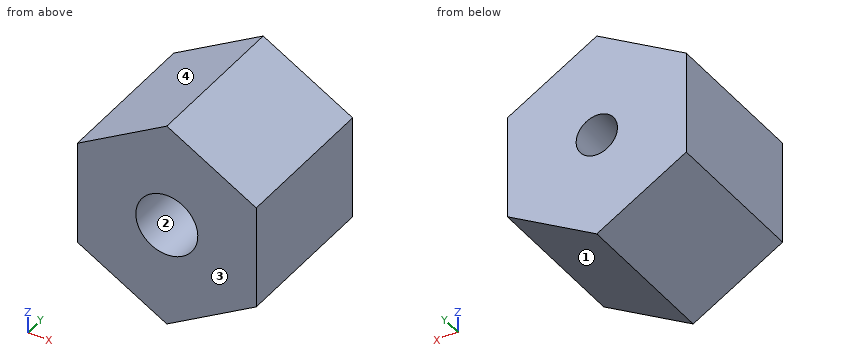
```python
from build123d import *

# Parameters (mm, degrees)
SKETCH2_R           = 2
BOSS_EXTRUDE1_DEPTH = 15
SKETCH2_4_R         = 3
CUT_EXTRUDE1_DEPTH  = 9


with BuildPart() as part:
    # Sketch2 → Boss-Extrude1 (new body)
    with BuildSketch(Plane(origin=(0, 0, 0), x_dir=(1, 0, 0), z_dir=(0, 1, 0))):
        Polygon((0, 10), (-8.660254038, 5), (-8.660254038, -5), (0, -10), (8.660254038, -5), (8.660254038, 5), align=None)
        with Locations(Location((0, 0, 0), (0, 0, 270))):
            Circle(SKETCH2_R, mode=Mode.SUBTRACT)
    extrude(amount=BOSS_EXTRUDE1_DEPTH)

    # Sketch2_4 → Cut-Extrude1 (cut)
    with BuildSketch(Plane(origin=(0, 0, 0), x_dir=(1, 0, 0), z_dir=(0, 1, 0))):
        with Locations(Location((0, 0, 0), (0, 0, 270))):
            Circle(SKETCH2_4_R)
    extrude(amount=CUT_EXTRUDE1_DEPTH, mode=Mode.SUBTRACT)


solid = part.part
```
Build history of the part. All positions in model axes, mm. Face numbers are marked on the shaded views. Coordinates: 2 decimals unless noted, no trailing zeros. Write each loop counter-clockwise with the first axis right and the second up, starting at its lowest first coordinate (ties: lowest second). Pieces come first, ordered by that corner, then holes.
1. Drop flat-ended pins along their axis: pin 1 (1.5 mm diameter, centred on x = -6.5, y = 6.5, fed in from -Z); pin 2 (3 mm diameter, centred on x = -3, y = 13, fed in from -Z); pin 3 (4 mm diameter, centred on x = -1, y = 7, fed in from +Z). Give the stop position or say it passes through.
Answer block:
pin 1: stops at z = -6.68
pin 2: stops at z = -9.13
pin 3: stops at z = 10
2. Drill centre lines: probe 1 along X at (y, z) = (10.9, 0); probe 2 along X at (y, z) = (2, 0); probe 3 along Z at (x, y) = (1.5, 11). Where is each one in solid material? Low to high.
Answer block:
probe 1: x = -8.66 to -2, 2 to 8.66
probe 2: x = -8.66 to -3, 3 to 8.66
probe 3: z = -9.13 to -1.32, 1.32 to 9.13
3. Pull direction X, two halves, no side cores. Call the marked faces 1, 2, 3 and 4: released by +X, released by -X, zero draft, split by the parting line, or undercut.
Answer block:
face 1: released by +X
face 2: undercut
face 3: zero draft
face 4: released by -X
4. Band-saw the part on D-D, the plane y = 7. Give the cut face in (x, z).
Answer block:
outline: (-8.66, -5) - (0, -10) - (8.66, -5) - (8.66, 5) - (0, 10) - (-8.66, 5) - close; hole circle Ø6 at (0, 0)
5. Band-saw the part on B-B, the plane z = 0. Give the cut face in (x, y).
Answer block:
outline: (-8.66, 0) - (-3, 0) - (-3, 9) - (-2, 9) - (-2, 15) - (-8.66, 15) - close; (2, 9) - (3, 9) - (3, 0) - (8.66, 0) - (8.66, 15) - (2, 15) - close
6. Band-saw the part on C-C, the plane x = -1.25. Give the cut face in (y, z), and give its area (3 significant figures).
Answer block:
outline: (0, -9.28) - (15, -9.28) - (15, -1.56) - (9, -1.56) - (9, -2.73) - (0, -2.73) - close; (0, 2.73) - (9, 2.73) - (9, 1.56) - (15, 1.56) - (15, 9.28) - (0, 9.28) - close
area: 211 mm2
7. Band-saw the part on A-A, the plane y = 11. Give the cut face in (x, z).
Answer block:
outline: (-8.66, -5) - (0, -10) - (8.66, -5) - (8.66, 5) - (0, 10) - (-8.66, 5) - close; hole circle Ø4 at (0, 0)
